Input: part model. Units: mm. Frame: model coordinates. A direction names the side the tool comes from. Round coordinates to 2 decimals unless told otherwise and drop trailing zeros. Order: outer loops, then holes, each group sorted by start corner. A loop starts at its lowest first (then second) coordinate and runs counter-clockwise, first axis right, second up.
Item 1: First-contact query: pin 1 (5 mm diameter, centred on y = -2.5, z = -7, fed in from -X); pin 2 (5 mm diameter, centred on x = -2.5, z = 3, fed in from +Y); pin 3 (2 mm diameter, centred on y = -1, z = 2.5, fed in from -X); pin 4 (1.5 mm diameter, centred on x = 2.5, z = -3.5, fed in from -Y). Flat tips, straight axial feed; report the tip coordinate or a pass-through.
Item 2: Reachability of faces 1 (the flat face through (-0.1, -2.2, 0)), 2 (the flat face through (0, 0, 5)) from +Z, -Z, +X, -X, +Y, -Y: full face, straight path, thin tool, end or side. Return the list, or none.
Item 3: Cut plane B-B on z = 1.25. Output: boundary loops of the cut face in (x, y), then the cut area to 3 significant figures.
Item 4: Cut plane A-A on z = -6.5. Output: boundary loops of the cut face in (x, y), then the cut area to 3 significant figures.
Item 5: Line query: L1, parallel to Y at x = -1, z = 2; L2, parallel to Y at x = 1.75, z = -9.25; L3, parallel to Z at x = -1, y = -4.25. Output: solid intervals per line, ascending.
```python
from build123d import *

# Parameters (mm, degrees)
SKETCH_R     = 2
PAD_DEPTH    = 5
SKETCH001_R  = 5
PAD001_DEPTH = 10
FILLET_R     = 3


with BuildPart() as part:
    # Sketch → Pad (new body)
    with BuildSketch(Plane.XY):
        Circle(SKETCH_R)
    extrude(amount=PAD_DEPTH)

    # Sketch001 → Pad001 (join)
    with BuildSketch(Plane.XY):
        Circle(SKETCH001_R)
    extrude(amount=-PAD001_DEPTH)

    # Fillet
    fillet_edges = [part.edges().sort_by_distance(p)[0] for p in [
        (-5, 0, -10),
    ]]
    fillet(fillet_edges, radius=FILLET_R)


solid = part.part
```
From the geometry:
1. pin 1: stops at x = -5
1. pin 2: stops at y = 2
1. pin 3: stops at x = -2
1. pin 4: stops at y = -4.68
2. face 1: +Z
2. face 2: +Z, +X, -X, +Y, -Y
3. outline: circle Ø4 at (0, 0)
3. area: 12.6 mm2
4. outline: circle Ø10 at (0, 0)
4. area: 78.5 mm2
5. L1: y = -1.73 to 1.73
5. L2: y = -3.58 to 3.58
5. L3: z = -8.84 to 0
